Part model, mm, in its own coordinate system. Face numbers are marked on the shaded views. A direction names the side the tool comes from. Round coordinates to 2 decimals unless told otherwise and drop trailing zeros. Write each loop counter-clockwise with the first axis right and the second up, starting at its lowest first coordinate (ties: lowest second). Pieces come first, ordered by that corner, then holes. Notation, with made-up numbers: M -18.5,84.5 L 31.5,84.5 A20 cw 31.5,109.5 Z; hole C 38,-26 d5. An arc over 180 degrees is marked long. One line per question, with ' | ' between items. Start each with the question number.
1) Wall check: probe 1 along Y at (x, z) = (-39.5, 22); probe 2 along Z at (x, y) = (-29, -56.5); probe 3 along Y at (x, z) = (-39, 15.75). Give the ranges that are in metal, low to high. Write a range as [from, to].
2) Saw through at D-D (y = -71.5). List the corners of the cut face in (x, z), plus the area to 3 significant figures.
3) Tool access for the marked faces 1, 2, 3 and 4: list every direction of +Z, -Z, +X, -X, +Y, -Y with a clear straight run to the whole face (end or side of a thin tool).
4) Saw through at B-B (x = -51.5). List the corners of the cut face in (y, z).
5) Drop flat-ended pins along their axis: pin 1 Ø2.5 at (x, z) = (-40, 7) entering from -Y; pin 2 Ø5 at (y, z) = (-29.5, 3.5) entering from -X; pin 3 Ø8 at (x, y) = (-28, -52) entering from +Z. Give the stop position or say it passes through.
6) Saw through at C-C (y = -57.5). List the corners of the cut face in (x, z), plus the area to 3 significant figures.
7) Saw through at A-A (y = -43.5). List the corners of the cut face in (x, z).
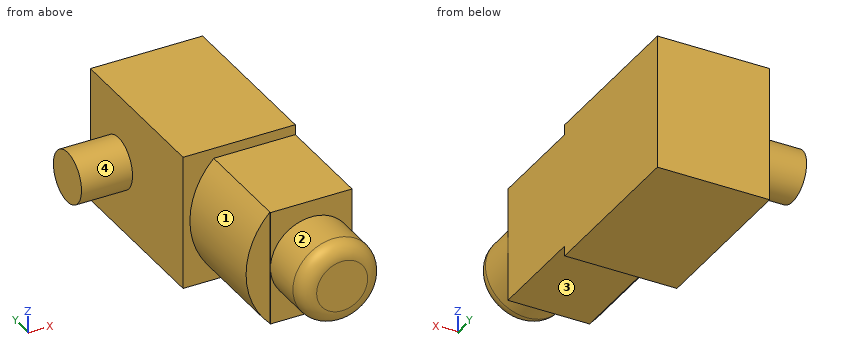
```python
from build123d import *

# Parameters (mm, degrees)
ESBO_O1_W                = 20
ESBO_O1_H                = 64.2
RESSALTO_EXTRUS_O1_DEPTH = 22.5
ESBO_O2_W                = 22.5
ESBO_O2_H                = 32.994304237
RESSALTO_EXTRUS_O2_DEPTH = 2
ESBO_O3_W                = 22
ESBO_O3_H                = 32.994304237
RESSALTO_EXTRUS_O3_DEPTH = 2
ESBO_O4_W                = 22
ESBO_O4_H                = 32.994304237
RESSALTO_EXTRUS_O5_DEPTH = 2
ESBO_O5_W                = 22.5
ESBO_O5_H                = 31.205695763
CORTE_EXTRUS_O1_DEPTH    = 4
RESSALTO_EXTRUS_O6_DEPTH = 20
CORTE_EXTRUS_O2_DEPTH    = 11
FILETE1_R                = 3
ESBO_O10_R               = 5
RESSALTO_EXTRUS_O7_DEPTH = 10


with BuildPart() as part:
    # Esboço1 → Ressalto-extrusão1 (new body)
    with BuildSketch(Plane.XY):
        with Locations((-32.828798315, -45.771841795)):
            Rectangle(ESBO_O1_W, ESBO_O1_H)
    extrude(amount=RESSALTO_EXTRUS_O1_DEPTH)

    # Esboço2 → Ressalto-extrusão2 (add)
    with BuildSketch(Plane.ZY.offset(42.828798315)):
        with Locations((11.25, -30.168993913)):
            Rectangle(ESBO_O2_W, ESBO_O2_H)
    extrude(amount=RESSALTO_EXTRUS_O2_DEPTH)

    # Esboço3 → Ressalto-extrusão3 (add)
    with BuildSketch(Plane(origin=(0, 0, 0), x_dir=(-1, 0, 0), z_dir=(0, 0, -1))):
        with Locations((33.828798315, -30.168993913)):
            Rectangle(ESBO_O3_W, ESBO_O3_H)
    extrude(amount=RESSALTO_EXTRUS_O3_DEPTH)

    # Esboço4 → Ressalto-extrusão5 (add)
    with BuildSketch(Plane.XY.offset(22.5)):
        with Locations((-33.828798315, -30.168993913)):
            Rectangle(ESBO_O4_W, ESBO_O4_H)
    extrude(amount=RESSALTO_EXTRUS_O5_DEPTH)

    # Esboço5 → Corte-extrusão1 (cut)
    with BuildSketch(Plane.ZY.offset(42.828798315)):
        with Locations((11.25, -62.268993914)):
            Rectangle(ESBO_O5_W, ESBO_O5_H)
    extrude(amount=-CORTE_EXTRUS_O1_DEPTH, mode=Mode.SUBTRACT)

    # Esboço8 → Ressalto-extrusão6 (add)
    with BuildSketch(Plane.XZ.offset(46.666146032)):
        with BuildLine():
            Line((-38.828798315, 0), (-38.828798315, 22.5))
            ThreePointArc((-38.828798315, 22.5), (-43.488700892, 11.25), (-38.828798315, 0))
        make_face()
    extrude(amount=RESSALTO_EXTRUS_O6_DEPTH)

    # Esboço9 → Corte-extrusão2 (cut)
    with BuildSketch(Plane(origin=(0, -77.871841795, 0), x_dir=(-1, 0, 0), z_dir=(0, -1, 0))):
        with BuildLine():
            Line((38.828798315, -22.5), (38.828798315, -11.25))
            ThreePointArc((38.828798315, -11.25), (30.828798315, -19.25), (22.828798315, -11.25))
            Line((22.828798315, -11.25), (22.828798315, -22.5))
            Line((22.828798315, -22.5), (38.828798315, -22.5))
        make_face()
        with BuildLine():
            Line((38.828798315, -11.25), (38.828798315, 0))
            Line((38.828798315, 0), (22.828798315, 0))
            Line((22.828798315, 0), (22.828798315, -11.25))
            ThreePointArc((22.828798315, -11.25), (30.828798315, -3.25), (38.828798315, -11.25))
        make_face()
    extrude(amount=-CORTE_EXTRUS_O2_DEPTH, mode=Mode.SUBTRACT)

    # Filete1
    filete1_edges = [part.edges().sort_by_distance(p)[0] for p in [
        (-22.828798315, -77.871841795, 11.25),
    ]]
    fillet(filete1_edges, radius=FILETE1_R)

    # Esboço10 → Ressalto-extrusão7 (add)
    with BuildSketch(Plane.ZY.offset(44.828798315)):
        with Locations(Location((11, -23.671841795, 0), (0, 0, 90))):
            Circle(ESBO_O10_R)
    extrude(amount=RESSALTO_EXTRUS_O7_DEPTH)


solid = part.part
```
Answer key:
1) probe 1: y = [-46.67, -13.67] | probe 2: z = [0, 22.5] | probe 3: y = [-66.67, -13.67]
2) outline: C -30.83,11.25 d16 | area: 201 mm2
3) face 1: -X, -Y | face 2: -Y | face 3: -Z, +X, -X, -Y | face 4: -X
4) outline: C -23.67,11 d10
5) pin 1: stops at y = -66.87 | pin 2: stops at x = -44.83 | pin 3: stops at z = 22.5
6) outline: M -38.83,0 L -22.83,0 L -22.83,22.5 L -38.83,22.5 A15.91 ccw Z | area: 432 mm2
7) outline: M -44.83,-2 L -22.83,-2 L -22.83,24.5 L -44.83,24.5 Z
